Study the drawing (mm; zero at the part's minimum x, y, z) and answer. A direction names the side the tool comes from. Coordinates: 2 decimals unless noted, no trailing zeros. Loops run counter-clockwise (first coordinate to the right, second up) from the corner with the lowest first, then second, coordinate; pieces in that order, holes last. Notation, with made-up numbers: (4, -12.75) - (11, -12.75) arc R28 ccw to (11, 26.25) - close; hole circle Ø1 at (-29, 83). An arc over 180 degrees is marked (long way). Put each result on its own line as item: value.
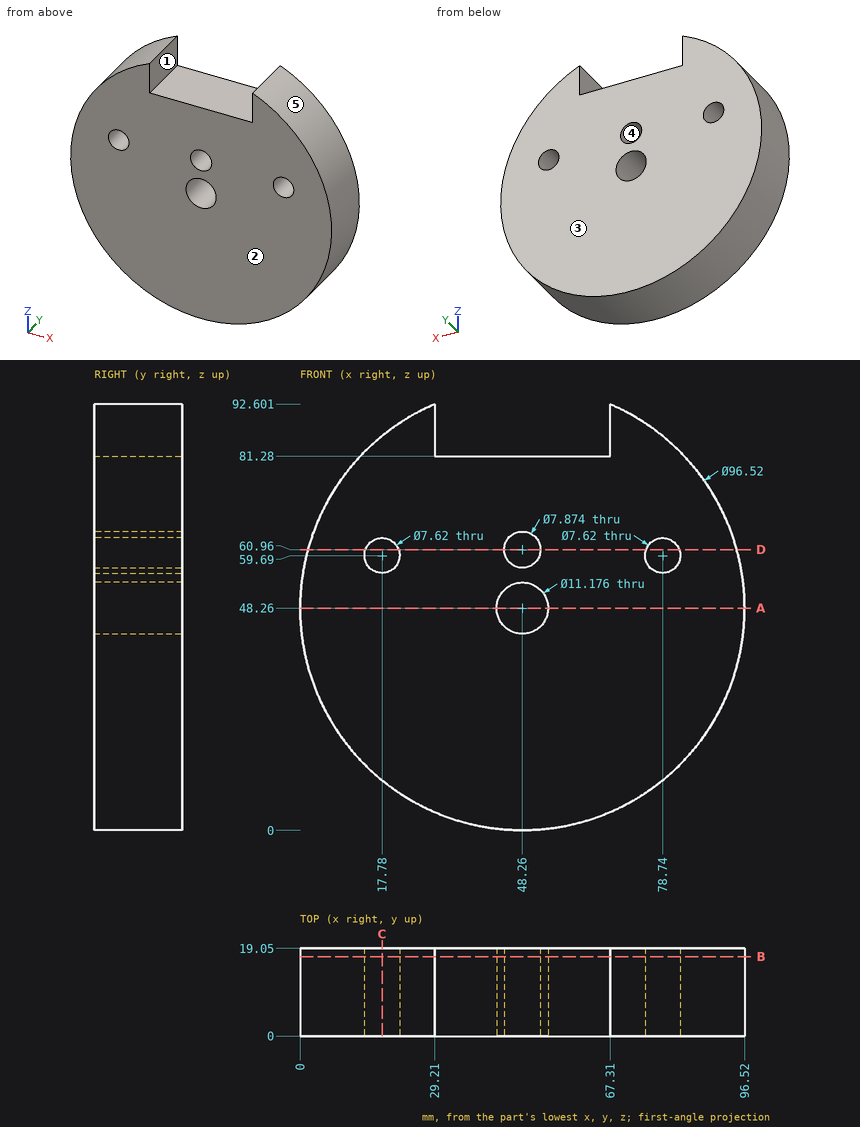
1) The part is cut by section D-D (z = 60.96). Give the vertices of the cut face in (x, y).
Found:
outline: (1.7, 0) - (14.19, 0) - (14.19, 19.05) - (1.7, 19.05) - close; (21.37, 0) - (44.32, 0) - (44.32, 19.05) - (21.37, 19.05) - close; (52.2, 0) - (75.15, 0) - (75.15, 19.05) - (52.2, 19.05) - close; (82.33, 0) - (94.82, 0) - (94.82, 19.05) - (82.33, 19.05) - close
2) The part is cut by section A-A (z = 48.26). Give the vertices of the cut face in (x, y).
Found:
outline: (0, 0) - (42.67, 0) - (42.67, 19.05) - (0, 19.05) - close; (53.85, 0) - (96.52, 0) - (96.52, 19.05) - (53.85, 19.05) - close
3) For a pull along Z with two mould halves and no side action, classify the marked faces 3, 4 and 5 as pulls with the +Z half, pulls with the -Z half, needs draft (parallel to the pull), parting line crosses it, or undercut.
Found:
face 3: needs draft
face 4: undercut
face 5: parting line crosses it
4) Straight lines are drawn through the part: L1, parallel to Z at x = 47, y = 17.25; L2, parallel to Z at x = 50, y = 7; L3, parallel to X at y = 9, z = 59.69. For each, find the intervals that lie inside material, in ascending order. Write a range as [from, to].
Found:
L1: z = [0.02, 42.82], [53.7, 57.23], [64.69, 81.28]
L2: z = [0.03, 42.95], [53.57, 57.43], [64.49, 81.28]
L3: x = [1.37, 13.97], [21.59, 44.53], [51.99, 74.93], [82.55, 95.15]
5) The part is cut by section B-B (y = 17.25). Give the vertices of the cut face in (x, z), and give its area (3 significant figures).
Found:
outline: (29.21, 81.28) - (29.21, 92.6) arc R48.26 ccw (long way) to (67.31, 92.6) - (67.31, 81.28) - close; hole circle Ø7.62 at (17.78, 59.69); hole circle Ø11.18 at (48.26, 48.26); hole circle Ø7.87 at (48.26, 60.96); hole circle Ø7.62 at (78.74, 59.69)
area: 6,550 mm^2
6) The part is cut by section C-C (x = 17.78). Give the vertices of the cut face in (y, z).
Found:
outline: (0, 10.84) - (19.05, 10.84) - (19.05, 55.88) - (0, 55.88) - close; (0, 63.5) - (19.05, 63.5) - (19.05, 85.68) - (0, 85.68) - close
7) For the marked faces 1 and 2, determine the directions among +Z, -Z, +X, -X, +Y, -Y from which every point of the face is accessible in a straight line to the end or side of a thin tool.
Found:
face 1: +Z, +Y, -Y
face 2: +Z, -Z, +X, -X, -Y
8) Each of these flat-tipped pins is pushed along its axis until it touches: pin 1 (5 mm diameter, centred on y = 4, z = 79, fed in from -X); pin 2 (2 mm diameter, centred on x = 13.5, y = 14.5, fed in from +Z); pin 3 (7 mm diameter, centred on x = 48.26, z = 60.96, fed in from -Y); pin 4 (3 mm diameter, centred on x = 54.5, y = 2.5, fed in from -Z). Where does it stop, or does it pass through?
Found:
pin 1: stops at x = 9.13
pin 2: stops at z = 82.75
pin 3: passes through
pin 4: stops at z = 0.23
